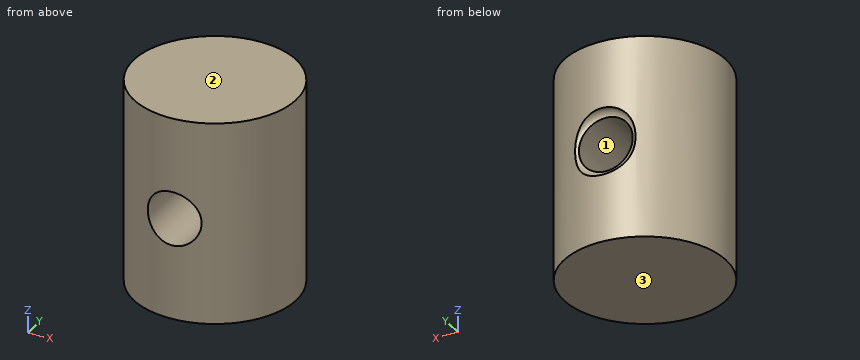
```python
from build123d import *

# Parameters (mm, degrees)
SZKIC1_R                    = 12
DODANIE_WYCI_GNI_CIE1_DEPTH = 15
OTW_R_8_0_8_1_D             = 8
SZKIC5_R                    = 1


with BuildPart() as part:
    # Szkic1 → Dodanie-wyci_gni_cie1 (new body, symmetric)
    with BuildSketch(Plane.XY):
        Circle(SZKIC1_R)
    extrude(amount=DODANIE_WYCI_GNI_CIE1_DEPTH, both=True)

    # Otw_r _8.0 _8_1 (through all)
    with Locations(Plane(origin=(0, 12, 0), x_dir=(1, 0, 0), z_dir=(0, 1, 0))):
        with Locations((0, 0)):
            Hole(OTW_R_8_0_8_1_D / 2)

    # Szkic5 → Wyci_cie-obr_t1 (revolve, cut)
    with BuildSketch(Plane(origin=(0, 0, 0), x_dir=(0, 0, -1), z_dir=(1, 0, 0))):
        with Locations((-4, 12)):
            Circle(SZKIC5_R)
    revolve(axis=Axis((0, -12, 0), (0, 1, 0)), mode=Mode.SUBTRACT)


solid = part.part
```
Geometry check sheet. Reference: the model listing, model coordinates, mm. Face numbers are marked on the shaded views. Give positions to 0.01 mm unless a question says otherwise; leave off trailing zeros. Loops run counter-clockwise (first coordinate to the right, second up) from the corner with the lowest first, then second, coordinate; pieces in that order, holes last. Notation, with made-up numbers: M 53,-23 L 89,-23 A14 cw 89,-5 Z; hole C 14.5,-5 d6. An arc over 180 degrees is marked long. Answer as CSV lines item,"result".
Item 1: Material ranges on line 1 (Z direction, x = -0.25, y = -4.75); line 2 (Z direction, x = -0.75, y = -5); line 3 (Y direction, x = 7.5, z = 12), recorded low to high.
Values:
line 1,"z = -15 to -3.99, 3.99 to 15"
line 2,"z = -15 to -3.93, 3.93 to 15"
line 3,"y = -9.37 to 9.37"
Item 2: Cross-section at D-D on z = -9. Record the cut outline in (x, y), and give its area (3 significant figures).
Values:
outline,"C 0,0 d24"
area,"452 mm²"
Item 3: Cross-section at A-A on x = 0. Record the cut outline in (y, z), and give its area (3 significant figures).
Values:
outline,"M -12,-15 L 12,-15 L 12,-5 A1 cw 11,-4 L -12,-4 Z; M -12,4 L 11,4 A1 cw 12,5 L 12,15 L -12,15 Z"
area,"526 mm²"
Item 4: Depth check by flat-ended pin: P1, Ø2, axis at y = 7, z = -4.5, coming from the -X side; P2, Ø2, axis at x = 5.5, z = 11, coming from the +Y side. Enter the tip coordinate at first touch or a pass-through.
Values:
P1,"stops at x = -10.39"
P2,"stops at y = 11.12"
Item 5: Cross-section at B-B on y = 0. Record the cut outline in (x, z).
Values:
outline,"M -12,-15 L 12,-15 L 12,15 L -12,15 Z; hole C 0,0 d8"
Item 6: Cross-section at C-C on z = 0. Record the cut outline in (x, y), and give its area (3 significant figures).
Values:
outline,"M -4.49,11.13 A12 ccw -4,-11.31 L -4,11 A1 cw Z; M 4,-11.31 A12 ccw 4.49,11.13 A1 cw 4,11 Z"
area,"264 mm²"
Item 7: Release check for a two-part mould opening along Z. For the marked faces 1, 2 and 3 record: pulls with the +Z half, pulls with the -Z half, needs draft (parallel to the pull), parting line crosses it, or undercut.
Values:
face 1,"undercut"
face 2,"pulls with the +Z half"
face 3,"pulls with the -Z half"
